Check sheet for the modelled part. Datum: model origin and axes. Units: mm. Face numbers are marked on the shaded views. A direction names the side the tool comes from. Coordinates: 2 decimals unless noted, no trailing zeros. Loops run counter-clockwise (first coordinate to the right, second up) from the corner with the lowest first, then second, coordinate; pieces in that order, holes last. Notation, with made-up numbers: (-8.5, 53.5) - (27.5, 53.5) arc R14 cw to (27.5, 57.5) - close; hole circle Ø3 at (79, -9.75). An arc over 180 degrees is marked (long way). Answer as a JSON object with one key per item and string values. Group by question number.
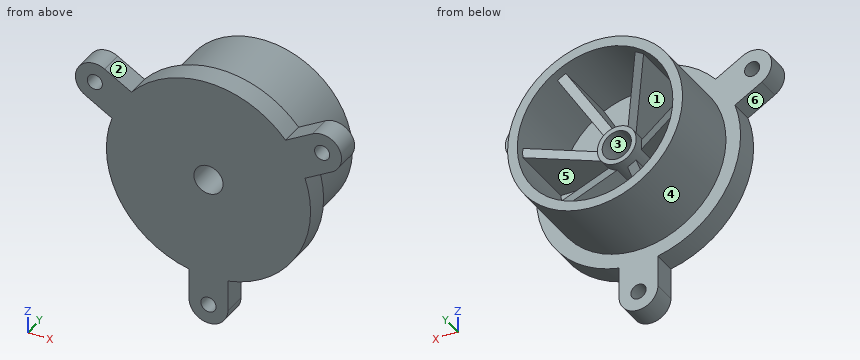
from build123d import *

# Parameters (mm, degrees)
SKETCH1_R           = 3.9
BOSS_EXTRUDE1_DEPTH = 12
SKETCH2_R           = 7.5
CUT_EXTRUDE1_DEPTH  = 12
BOSS_EXTRUDE2_START = 20
SKETCH4_R           = 10
SKETCH4_R_2         = 7.5
BOSS_EXTRUDE2_DEPTH = 20
SKETCH5_R           = 45
SKETCH5_R_2         = 40
BOSS_EXTRUDE3_DEPTH = 40
RIB1_START          = -2.5
RIB1_DEPTH          = 5
CIRPATTERN1_COUNT   = 6


# Read off the part's stored shape, not the designer's step: Rib1
with BuildPart() as part:
    # Sketch1 → Boss-Extrude1 (new body)
    with BuildSketch(Plane(origin=(0, 0, 0), x_dir=(1, 0, 0), z_dir=(0, 1, 0))):
        with BuildLine():
            ThreePointArc((10, 67.5), (0, 77.5), (-10, 67.5))
            Line((-10, 67.5), (-10, 51.53882032))
            ThreePointArc((-10, 51.53882032), (-45.466333699, 26.25), (-49.633927678, -17.109156122))
            Line((-49.633927678, -17.109156122), (-63.456714755, -25.089745962))
            ThreePointArc((-63.456714755, -25.089745962), (-67.116968793, -38.75), (-53.456714755, -42.410254038))
            Line((-53.456714755, -42.410254038), (-39.633927678, -34.429664198))
            ThreePointArc((-39.633927678, -34.429664198), (0, -52.5), (39.633927678, -34.429664198))
            Line((39.633927678, -34.429664198), (53.456714755, -42.410254038))
            ThreePointArc((53.456714755, -42.410254038), (67.116968793, -38.75), (63.456714755, -25.089745962))
            Line((63.456714755, -25.089745962), (49.633927678, -17.109156122))
            ThreePointArc((49.633927678, -17.109156122), (45.466333699, 26.25), (10, 51.53882032))
            Line((10, 51.53882032), (10, 67.5))
        make_face()
        with Locations(Location((-58.456714755, -33.75, 0), (0, 0, 270))):
            Circle(SKETCH1_R, mode=Mode.SUBTRACT)
        with Locations(Location((58.456714755, -33.75, 0), (0, 0, 270))):
            Circle(SKETCH1_R, mode=Mode.SUBTRACT)
        with Locations(Location((0, 67.5, 0), (0, 0, 270))):
            Circle(SKETCH1_R, mode=Mode.SUBTRACT)
    extrude(amount=BOSS_EXTRUDE1_DEPTH)

    # Sketch2 → Cut-Extrude1 (cut)
    with BuildSketch(Plane(origin=(0, 12, 0), x_dir=(1, 0, 0), z_dir=(0, 1, 0))):
        with Locations(Location((0, 0, 0), (0, 0, 270))):
            Circle(SKETCH2_R)
    extrude(amount=-CUT_EXTRUDE1_DEPTH, mode=Mode.SUBTRACT)

    # Sketch4 → Boss-Extrude2 (add)
    with BuildSketch(Plane(origin=(0, 12, 0), x_dir=(1, 0, 0), z_dir=(0, 1, 0)).offset(BOSS_EXTRUDE2_START)):
        with Locations(Location((0, 0, 0), (0, 0, 270))):
            Circle(SKETCH4_R)
        with Locations(Location((0, 0, 0), (0, 0, 270))):
            Circle(SKETCH4_R_2, mode=Mode.SUBTRACT)
    extrude(amount=-BOSS_EXTRUDE2_DEPTH)

    # Sketch5 → Boss-Extrude3 (add)
    with BuildSketch(Plane(origin=(0, 12, 0), x_dir=(1, 0, 0), z_dir=(0, 1, 0))):
        with Locations(Location((0, 0, 0), (0, 0, 270))):
            Circle(SKETCH5_R)
        with Locations(Location((0, 0, 0), (0, 0, 270))):
            Circle(SKETCH5_R_2, mode=Mode.SUBTRACT)
    extrude(amount=BOSS_EXTRUDE3_DEPTH)

    # Rib1 outline → Rib1 (add)
    with BuildSketch(Plane.XY.offset(RIB1_START)):
        Polygon((40, 47), (9.682458366, 26.788305577), (8, 25.666666666), (8, 12), (41, 12), (41, 47.666666667), align=None)
    rib1 = extrude(amount=RIB1_DEPTH)

    # CirPattern1: Rib1 ×6 about axis
    cirpattern1_axis = Axis((0, 0, 0), (0, 1, 0))
    for i in range(1, CIRPATTERN1_COUNT):
        add(rib1.rotate(cirpattern1_axis, i * 360 / CIRPATTERN1_COUNT))


solid = part.part
1. Sectioned sample at C-C on z = 0. Record the cut outline in (x, y), plus the area to 3 significant figures.
2. Sectioned sample at B-B on y = 25. Record the cut outline in (x, z).
3. Release check for a two-part mould opening along X. For the marked faces 4, 5 and 6 record: released by +X, released by -X, zero draft, split by the parting line, or undercut.
4. Material ranges on line 1 (X direction, y = 6, z = 33.75); line 2 (X direction, y = 43, z = 31); line 3 (Z direction, x = 34.5, y = 22.5), recorded low to high.
5. Sectioned sample at A-A on x = 0. Record the cut outline in (y, z).
6. Gauge pin test, flat ends, axial feed: pin 1 (24 mm diameter, centred on x = -18, y = 35.5, fed in from +Z); pin 2 (24 mm diameter, centred on x = 19, y = 25.5, fed in from -Z); pin 3 (1 mm diameter, centred on x = 32.5, y = 46.5, fed in from +Z). Record the tip position at first contact, or that the pin passes through.
7. Sectioned sample at D-D on y = 41. Record the cut outline in (x, z), plus the area to 3 significant figures.
8. Access from +Z, -Z, +X, -X, +Y, -Y to the whole of each face (thin tool, end or side, straight path). Record for the marked faces 1, 2 and 3.
Answers follow:
{
 "1": {"outline": "(-52.5, 0) - (-7.5, 0) - (-7.5, 32) - (-10, 32) - (-10, 27) - (-40, 47) - (-40, 52) - (-45, 52) - (-45, 12) - (-52.5, 12) - close; (7.5, 0) - (52.5, 0) - (52.5, 12) - (45, 12) - (45, 52) - (40, 52) - (40, 47) - (10, 27) - (10, 32) - (7.5, 32) - close", "area": "3,080 mm^2"},
 "2": {"outline": "circle Ø90 at (0, 0); hole (-39.92, -2.5) arc R40 ccw to (-22.13, -33.32) - (-7.01, -7.14) arc R10 cw to (-9.68, -2.5) - close; hole (-39.92, 2.5) - (-9.68, 2.5) arc R10 cw to (-7.01, 7.14) - (-22.13, 33.32) arc R40 ccw to start; hole (-17.8, -35.82) arc R40 ccw to (17.8, -35.82) - (2.68, -9.64) arc R10 cw to (-2.68, -9.64) - close; hole (-17.8, 35.82) - (-2.68, 9.64) arc R10 cw to (2.68, 9.64) - (17.8, 35.82) arc R40 ccw to start; hole circle Ø15 at (0, 0); hole (7.01, -7.14) - (22.13, -33.32) arc R40 ccw to (39.92, -2.5) - (9.68, -2.5) arc R10 cw to start; hole (7.01, 7.14) arc R10 cw to (9.68, 2.5) - (39.92, 2.5) arc R40 ccw to (22.13, 33.32) - close"},
 "3": {"face 4": "split by the parting line", "face 5": "undercut", "face 6": "released by -X"},
 "4": {"line 1": "x = -68.46 to -62.36, -54.56 to 54.56, 62.36 to 68.46", "line 2": "x = -32.62 to -25.28, -20.78 to -15.01, 15.01 to 20.78, 25.28 to 32.62", "line 3": "z = -28.89 to -20.24, -2.5 to 2.5, 20.24 to 28.89"},
 "5": {"outline": "(0, -77.5) - (12, -77.5) - (12, -71.4) - (0, -71.4) - close; (0, -63.6) - (12, -63.6) - (12, -45) - (52, -45) - (52, -40) - (12, -40) - (12, -10) - (32, -10) - (32, -7.5) - (0, -7.5) - close; (0, 7.5) - (32, 7.5) - (32, 10) - (12, 10) - (12, 40) - (52, 40) - (52, 45) - (12, 45) - (12, 52.5) - (0, 52.5) - close"},
 "6": {"pin 1": "stops at z = 44.6", "pin 2": "stops at z = -44.45", "pin 3": "stops at z = 31.64"},
 "7": {"outline": "circle Ø90 at (0, 0); hole (-39.92, -2.5) arc R40 ccw to (-22.13, -33.32) - (-17.67, -25.6) - (-13.33, -28.1) - (-17.8, -35.82) arc R40 ccw to (17.8, -35.82) - (13.33, -28.1) - (17.67, -25.6) - (22.13, -33.32) arc R40 ccw to (39.92, -2.5) - (31, -2.5) - (31, 2.5) - (39.92, 2.5) arc R40 ccw to (22.13, 33.32) - (17.67, 25.6) - (13.33, 28.1) - (17.8, 35.82) arc R40 ccw to (-17.8, 35.82) - (-13.33, 28.1) - (-17.67, 25.6) - (-22.13, 33.32) arc R40 ccw to (-39.92, 2.5) - (-31, 2.5) - (-31, -2.5) - close", "area": "1,600 mm^2"},
 "8": {"face 1": "+Y", "face 2": "+Z, +Y, -Y", "face 3": "+Y, -Y"}
}
